```python
from build123d import *

# Parameters (mm, degrees)
F0_W           = 75.8636072278
F0_H           = 76.6314566135
F1_DEPTH       = 76.2
F3_D           = 12.7
F3_DEPTH       = 38.1
F3_CBORE_D     = 25.4
F3_CBORE_DEPTH = 6.35
F3_TIP         = 3.8154649308
F5_D           = 12.7
F5_DEPTH       = 38.1
F5_CBORE_D     = 25.4
F5_CBORE_DEPTH = 6.35
F5_TIP         = 3.8154649308


with BuildPart() as f1:
    # F0 (on Right) → F1 (new body)
    with BuildSketch(Plane.YZ):
        with Locations((-37.9318036139, 38.3157283068)):
            Rectangle(F0_W, F0_H)
    extrude(amount=F1_DEPTH)

    # F3
    with Locations(Plane.XZ.offset(75.8636072278)):
        with Locations((36.8568152189, 40.0817841291)):
            CounterBoreHole(F3_D / 2, F3_CBORE_D / 2, F3_CBORE_DEPTH, depth=F3_DEPTH)
            with Locations((0, 0, -(F3_DEPTH + F3_TIP / 2))):  # 118° drill point
                Cone(0, F3_D / 2, F3_TIP, mode=Mode.SUBTRACT)

    # F5
    with Locations(Plane.YZ.offset(76.2)):
        with Locations((-38.6996529996, 39.1603671014)):
            CounterBoreHole(F5_D / 2, F5_CBORE_D / 2, F5_CBORE_DEPTH, depth=F5_DEPTH)
            with Locations((0, 0, -(F5_DEPTH + F5_TIP / 2))):  # 118° drill point
                Cone(0, F5_D / 2, F5_TIP, mode=Mode.SUBTRACT)


solid = f1.part
```
Could you check a few things on this model? Use its own coordinates, in mm. A direction names the side the tool comes from. Give positions to 0.01 mm unless a question says otherwise; leave off trailing zeros. Loops run counter-clockwise (first coordinate to the right, second up) from the corner with the lowest first, then second, coordinate; pieces in that order, holes last. Notation, with made-up numbers: (-36, -16.5) - (-13, -16.5) arc R22 cw to (-13, 6.5) - close; hole circle Ø8 at (21.5, 87.25). An arc over 180 degrees is marked (long way). Use one line per item in the form item = value.
1. I need wall thicknesses on probe 1 along Z at (x, y) = (65, -36.5); probe 2 along X at (y, z) = (-71.5, 32); probe 3 along Z at (x, y) = (33, -52.5). Which ranges of each line are inside material? Lowest first, please.
Response values:
probe_1 = 0 to 33.2, 45.12 to 76.63
probe_2 = 0 to 27.06, 46.65 to 76.2
probe_3 = 0 to 35.04, 45.13 to 76.63
2. I'm going to push a flat-ended pin straight in: pin 1 Ø7.5 at (y, z) = (-38.7, 39.16) entering from +X. Where does the tip first touch, or does it pass through?
Response values:
pin_1 = 36.54
3. Thinking about a two-plate mould opening in Z: for faces 1 (the face through (76.2, -55, 39)), 2 (the face through (36.725, -35.016, 37.447)), 3 (the face through (30.8, -53.42, 41.99)), 4 (the face through (38, -38, 0)), which applies, released by +Z, released by -Z, zero draft, split by the parting line, or undercut?
Response values:
face_1 = zero draft
face_2 = undercut
face_3 = undercut
face_4 = released by -Z
4. I want a section at A-A (y = -63.5). Please give me the cut outline in (x, z).
Response values:
outline = (0, 0) - (76.2, 0) - (76.2, 76.63) - (0, 76.63) - close; hole circle Ø12.7 at (36.86, 40.08)
5. On a 3-axis mill with a long thin cutter (end or side, diameter ignored), from which of +Z, -Z, +X, -X, +Y, -Y can I reach the whole of each face in a straight line? I mean faces 5 (the face through (69.85, -45, 37)), 6 (the face through (46, -75.864, 29)), 7 (the face through (31, -69.514, 37)). Say none if no direction works.
Response values:
face_5 = +X
face_6 = +Z, -Z, +X, -X, -Y
face_7 = -Y
